from build123d import *

# Parameters (mm, degrees)
BOSS_EXTRUDE1_DEPTH                   = 9
BOSS_EXTRUDE1_DEPTH_BACK              = 9
TAP_DRILL_FOR_M4_TAP1_D               = 3.3
TAP_DRILL_FOR_M4_TAP1_DEPTH           = 25
TAP_DRILL_FOR_M4_TAP1_TIP             = 0.991420021
TAP_DRILL_FOR_M4_TAP1_ON_FACE_2_D     = 3.3
TAP_DRILL_FOR_M4_TAP1_ON_FACE_2_DEPTH = 25
TAP_DRILL_FOR_M4_TAP1_ON_FACE_2_TIP   = 0.991420021
TAP_DRILL_FOR_M4_TAP1_ON_FACE_3_D     = 3.3
TAP_DRILL_FOR_M4_TAP1_ON_FACE_3_DEPTH = 25
TAP_DRILL_FOR_M4_TAP1_ON_FACE_3_TIP   = 0.991420021
TAP_DRILL_FOR_M4_TAP1_ON_FACE_4_D     = 3.3
TAP_DRILL_FOR_M4_TAP1_ON_FACE_4_DEPTH = 25
TAP_DRILL_FOR_M4_TAP1_ON_FACE_4_TIP   = 0.991420021
TAP_DRILL_FOR_M4_TAP1_ON_FACE_5_D     = 3.3
TAP_DRILL_FOR_M4_TAP1_ON_FACE_5_DEPTH = 25
TAP_DRILL_FOR_M4_TAP1_ON_FACE_5_TIP   = 0.991420021
TAP_DRILL_FOR_M4_TAP1_ON_FACE_6_D     = 3.3
TAP_DRILL_FOR_M4_TAP1_ON_FACE_6_DEPTH = 25
TAP_DRILL_FOR_M4_TAP1_ON_FACE_6_TIP   = 0.991420021
FILLET2_R                             = 2
CUT_EXTRUDE2_DEPTH                    = 159.865224489
CUT_EXTRUDE2_DEPTH_BACK               = 159.865224489
SKETCH3_R                             = 5
FILLET3_R                             = 1.5
BOSS_EXTRUDE2_START                   = 9
BOSS_EXTRUDE2_DEPTH                   = 30
FILLET4_R                             = 1.5
FILLET5_R                             = 2
CUT_EXTRUDE3_DEPTH                    = 164.257977095
CUT_EXTRUDE3_DEPTH_BACK               = 164.257977095
SKETCH4_3_R                           = 3
FILLET6_R                             = 1.5
WRAP1_START                           = -0.5
WRAP1_DEPTH                           = 0.5


# Read off the part's stored shape, not the designer's step: Wrap1
with BuildPart() as part:
    # Sketch1 → Boss-Extrude1 (new, two sides: drawn at the far end of the back side and taken through both)
    with BuildSketch(Plane.XY.offset(-BOSS_EXTRUDE1_DEPTH_BACK)):
        with BuildLine():
            Line((66.491800306, -127.729559978), (66.491800306, -83.193091613))
            ThreePointArc((66.491800306, -83.193091613), (0, -106.5), (-66.491800306, -83.193091613))
            Line((-66.491800306, -83.193091613), (-66.491800306, -127.729559978))
            ThreePointArc((-66.491800306, -127.729559978), (0, -144), (66.491800306, -127.729559978))
        make_face()
    extrude(amount=BOSS_EXTRUDE1_DEPTH + BOSS_EXTRUDE1_DEPTH_BACK)

    # Tap Drill for M4 Tap1
    with Locations(Plane(origin=(-32.025167647, -101.570855255, 0), x_dir=(0.953716950748, -0.300705799504, 0), z_dir=(0.300705799504, 0.953716950748, 0))):
        with Locations((0, 0)):
            Hole(TAP_DRILL_FOR_M4_TAP1_D / 2, depth=TAP_DRILL_FOR_M4_TAP1_DEPTH)
            with Locations((0, 0, -(TAP_DRILL_FOR_M4_TAP1_DEPTH + TAP_DRILL_FOR_M4_TAP1_TIP / 2))):  # 118° drill point
                Cone(0, TAP_DRILL_FOR_M4_TAP1_D / 2, TAP_DRILL_FOR_M4_TAP1_TIP, mode=Mode.SUBTRACT)

    # Tap Drill for M4 Tap1 on face 2
    with Locations(Plane(origin=(32.025167647, -101.570855255, 0), x_dir=(0.953716897702, 0.300705967746, 0), z_dir=(-0.300705967746, 0.953716897702, 0))):
        with Locations((0, 0)):
            Hole(TAP_DRILL_FOR_M4_TAP1_ON_FACE_2_D / 2, depth=TAP_DRILL_FOR_M4_TAP1_ON_FACE_2_DEPTH)
            with Locations((0, 0, -(TAP_DRILL_FOR_M4_TAP1_ON_FACE_2_DEPTH + TAP_DRILL_FOR_M4_TAP1_ON_FACE_2_TIP / 2))):  # 118° drill point
                Cone(0, TAP_DRILL_FOR_M4_TAP1_ON_FACE_2_D / 2, TAP_DRILL_FOR_M4_TAP1_ON_FACE_2_TIP, mode=Mode.SUBTRACT)

    # Tap Drill for M4 Tap1 on face 3
    with Locations(Plane(origin=(-55.106414261, -133.038652682, 0), x_dir=(-0.923879753837, 0.382682898036, 0), z_dir=(-0.382682898036, -0.923879753837, 0))):
        with Locations((0, 0)):
            Hole(TAP_DRILL_FOR_M4_TAP1_ON_FACE_3_D / 2, depth=TAP_DRILL_FOR_M4_TAP1_ON_FACE_3_DEPTH)
            with Locations((0, 0, -(TAP_DRILL_FOR_M4_TAP1_ON_FACE_3_DEPTH + TAP_DRILL_FOR_M4_TAP1_ON_FACE_3_TIP / 2))):  # 118° drill point
                Cone(0, TAP_DRILL_FOR_M4_TAP1_ON_FACE_3_D / 2, TAP_DRILL_FOR_M4_TAP1_ON_FACE_3_TIP, mode=Mode.SUBTRACT)

    # Tap Drill for M4 Tap1 on face 4
    with Locations(Plane(origin=(18.79577168, -142.768060038, 0), x_dir=(-0.991444888611, -0.130525985335, 0), z_dir=(0.130525985335, -0.991444888611, 0))):
        with Locations((0, 0)):
            Hole(TAP_DRILL_FOR_M4_TAP1_ON_FACE_4_D / 2, depth=TAP_DRILL_FOR_M4_TAP1_ON_FACE_4_DEPTH)
            with Locations((0, 0, -(TAP_DRILL_FOR_M4_TAP1_ON_FACE_4_DEPTH + TAP_DRILL_FOR_M4_TAP1_ON_FACE_4_TIP / 2))):  # 118° drill point
                Cone(0, TAP_DRILL_FOR_M4_TAP1_ON_FACE_4_D / 2, TAP_DRILL_FOR_M4_TAP1_ON_FACE_4_TIP, mode=Mode.SUBTRACT)

    # Tap Drill for M4 Tap1 on face 5
    with Locations(Plane(origin=(55.106414261, -133.038652682, 0), x_dir=(-0.923879753837, -0.382682898036, 0), z_dir=(0.382682898036, -0.923879753837, 0))):
        with Locations((0, 0)):
            Hole(TAP_DRILL_FOR_M4_TAP1_ON_FACE_5_D / 2, depth=TAP_DRILL_FOR_M4_TAP1_ON_FACE_5_DEPTH)
            with Locations((0, 0, -(TAP_DRILL_FOR_M4_TAP1_ON_FACE_5_DEPTH + TAP_DRILL_FOR_M4_TAP1_ON_FACE_5_TIP / 2))):  # 118° drill point
                Cone(0, TAP_DRILL_FOR_M4_TAP1_ON_FACE_5_D / 2, TAP_DRILL_FOR_M4_TAP1_ON_FACE_5_TIP, mode=Mode.SUBTRACT)

    # Tap Drill for M4 Tap1 on face 6
    with Locations(Plane(origin=(-18.79577168, -142.768060038, 0), x_dir=(-0.991444888611, 0.130525985335, 0), z_dir=(-0.130525985335, -0.991444888611, 0))):
        with Locations((0, 0)):
            Hole(TAP_DRILL_FOR_M4_TAP1_ON_FACE_6_D / 2, depth=TAP_DRILL_FOR_M4_TAP1_ON_FACE_6_DEPTH)
            with Locations((0, 0, -(TAP_DRILL_FOR_M4_TAP1_ON_FACE_6_DEPTH + TAP_DRILL_FOR_M4_TAP1_ON_FACE_6_TIP / 2))):  # 118° drill point
                Cone(0, TAP_DRILL_FOR_M4_TAP1_ON_FACE_6_D / 2, TAP_DRILL_FOR_M4_TAP1_ON_FACE_6_TIP, mode=Mode.SUBTRACT)

    # Fillet2
    fillet2_edges = [part.edges().sort_by_distance(p)[0] for p in [
        (66.491800306, -83.193091613, 0),
        (-66.491800306, -83.193091613, 0),
    ]]
    fillet(fillet2_edges, radius=FILLET2_R)

    # Sketch3 → Cut-Extrude2 (cut, two sides: drawn at the far end of the back side and taken through both)
    with BuildSketch(Plane.XY.offset(-CUT_EXTRUDE2_DEPTH_BACK)):
        with Locations((0, -144)):
            Circle(SKETCH3_R)
    extrude(amount=CUT_EXTRUDE2_DEPTH + CUT_EXTRUDE2_DEPTH_BACK, mode=Mode.SUBTRACT)

    # Fillet3
    fillet3_edges = [part.edges().sort_by_distance(p)[0] for p in [
        (0, -139, -9),
        (0, -139, 9),
    ]]
    fillet(fillet3_edges, radius=FILLET3_R)

    # Sketch4 → Boss-Extrude2 (add)
    with BuildSketch(Plane.XY.offset(BOSS_EXTRUDE2_START)):
        with BuildLine():
            Line((0, -115.5), (0, -111.5))
            ThreePointArc((0, -111.5), (-7.517102754, -111.24631754), (-15, -110.486424505))
            Line((-15, -110.486424505), (-15, -115.5))
            Line((-15, -115.5), (0, -115.5))
        make_face()
        with BuildLine():
            ThreePointArc((15, -110.486424505), (7.517102754, -111.24631754), (0, -111.5))
            Line((0, -111.5), (0, -115.5))
            Line((0, -115.5), (15, -115.5))
            Line((15, -115.5), (15, -110.486424505))
        make_face()
    extrude(amount=BOSS_EXTRUDE2_DEPTH)

    # Fillet4
    fillet4_edges = [part.edges().sort_by_distance(p)[0] for p in [
        (-15, -112.993212253, 9),
        (0, -111.5, 9),
        (15, -112.993212253, 9),
    ]]
    fillet(fillet4_edges, radius=FILLET4_R)

    # Fillet5
    # the kernel refuses this fillet: 2 mm, written as the material it takes off along each edge
    with BuildSketch(Plane(origin=(66.491800306, -132.729559978, -9), x_dir=(-1, 0, 0), z_dir=(0, 1, 0)), Plane(origin=(-66.491800306, -82.252837738, -9), x_dir=(1, 0, 0), z_dir=(0, -1, 0))) as fillet5_piece_1:
        with BuildLine():
            CenterArc((FILLET5_R, FILLET5_R), FILLET5_R, 180, 90)
            Line((0, FILLET5_R), (0, 0))
            Line((0, 0), (FILLET5_R, 0))
        make_face()
    extrude(amount=50.47672224, mode=Mode.SUBTRACT)

    # Sketch4<3> → Cut-Extrude3 (cut, two sides: drawn at the far end of the back side and taken through both)
    with BuildSketch(Plane.XY.offset(-CUT_EXTRUDE3_DEPTH_BACK)):
        with Locations((-8, -124.5)):
            Circle(SKETCH4_3_R)
        with Locations((8, -124.5)):
            Circle(SKETCH4_3_R)
    extrude(amount=CUT_EXTRUDE3_DEPTH + CUT_EXTRUDE3_DEPTH_BACK, mode=Mode.SUBTRACT)

    # Fillet6
    fillet6_edges = [part.edges().sort_by_distance(p)[0] for p in [
        (-11, -124.5, -9),
        (5, -124.5, -9),
    ]]
    fillet(fillet6_edges, radius=FILLET6_R)

    # Wrap1 outline → Wrap1 (cut)
    with BuildSketch(Plane(origin=(0, 0, -9), x_dir=(-1, 0, 0), z_dir=(0, 0, -1)).offset(WRAP1_START)):
        Polygon((-5.892307692, -130.820512821), (-5.892307692, -130), (-10.097435897, -130), (-10.097435897, -130.820512821), (-8.353846154, -130.820512821), (-8.353846154, -138), (-7.635897436, -138), (-7.635897436, -130.820512821), align=None)
        Polygon((7.976923077, -136.564102564), (4.674038462, -130), (4.571474359, -130), (3.515384615, -138), (4.238141026, -138), (5.002564103, -132.230769231), (7.901602564, -138), (8.063461538, -138), (10.951282051, -132.243589744), (11.717307692, -138), (12.438461538, -138), (11.375961538, -130), (11.271794872, -130), align=None)
    extrude(amount=WRAP1_DEPTH, mode=Mode.SUBTRACT)


solid = part.part
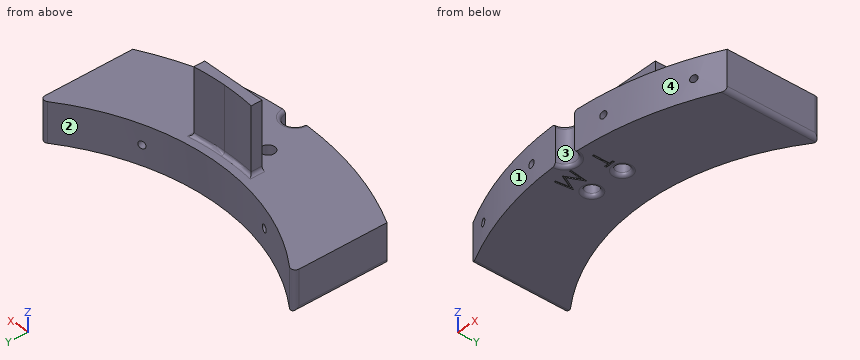
Work out the finished part from the listing and answer in its coordinate system (mm). Face numbers are marked on the shaded views. Give positions to 0.01 mm unless a question says otherwise; leave off trailing zeros. Order: outer loops, then holes, each group sorted by start corner. A loop starts at its lowest first (then second) coordinate and runs counter-clockwise, first axis right, second up. Notation, with made-up numbers: (-3.75, -24.5) -> (16.25, -24.5) arc R26 cw to (16.25, 2.5) -> close; hole circle Ø3 at (20, -27). An arc over 180 degrees is marked (long way). Answer as a JSON object with one key per item and string values. Group by question number.
1. The mould has two halves that part along X. Classify the marked faces 1, 2, 3 and 4: released by +X, released by -X, zero draft, split by the parting line, or undercut.
2. Flat-ended cylindrical pins translate along their axes: pin 1 Ø10 at (y, z) = (-99.5, 13.5) entering from -X; pin 2 Ø1 at (x, y) = (-41, -101.5) entering from +Z; pin 3 Ø0.6 at (y, z) = (-130.5, -8.5) entering from +X; pin 4 Ø7 at (x, y) = (-8, -124.5) entering from -Z. Find the tip coordinate at first contact, or state that the pin passes through.
3. Section B-B on z = 24 is taken. Determine the outline of the cut face in (x, y), plus the area to 3 significant figures.
4. Section A-A on y = -98 is taken. Determine the outline of the cut face in (x, z), plus the area to 3 significant figures.
5. Consider line 1 along X through (y, z) = (-124.5, -1.75); line 2 along Z through (x, y) = (-3, -133); line 3 along Y through (x, z) = (8, -3.5). Determine where each line is inside the solid, lowest interval first. Write a range as [from, to].
Result sheet:
{
 "1": {"face 1": "released by -X", "face 2": "undercut", "face 3": "undercut", "face 4": "released by +X"},
 "2": {"pin 1": "stops at x = -66.49", "pin 2": "stops at z = 9", "pin 3": "stops at x = 61.51", "pin 4": "stops at z = -8.62"},
 "3": {"outline": "(-15, -115.5) -> (15, -115.5) -> (15, -110.49) arc R111.5 cw to (-15, -110.49) -> close", "area": "130 mm^2"},
 "4": {"outline": "(-66.49, -7) arc R2 ccw to (-64.49, -9) -> (-41.69, -9) -> (-41.69, 9) -> (-66.49, 9) -> close; (41.69, -9) -> (64.49, -9) arc R2 ccw to (66.49, -7) -> (66.49, 9) -> (41.69, 9) -> close", "area": "891 mm^2"},
 "5": {"line 1": "x = [-66.49, -11], [-5, 5], [11, 66.49]", "line 2": "z = [-9, 9]", "line 3": "y = [-143.78, -127.5], [-121.5, -106.2]"}
}
